from build123d import *
from OCP.BRepFilletAPI import BRepFilletAPI_MakeChamfer

# Parameters (mm, degrees)
SKETCH1_W          = 20.1676
SKETCH1_H          = 40.2082
EXTRUDE1_DEPTH     = 26.4668
SKETCH2_W          = 20.1676
SKETCH2_H          = 40.2082
EXTRUDE2_DEPTH     = 2.4892
SKETCH3_W          = 20.1676
SKETCH3_H          = 40.2082
EXTRUDE3_DEPTH     = 4.445
SKETCH11_W         = 20.1676
SKETCH11_H         = 0.2667
CUT_EXTRUDE2_DEPTH = 4.445
EXTRUDE4_DEPTH     = 2.38125
SKETCH5_R          = 7.62
EXTRUDE5_DEPTH     = 2.57175
CHAMFER1_SIZE      = 2.54
CHAMFER1_SIZE2     = 1.466469684
EXTRUDE6_DEPTH     = 0.635
SKETCH8_R          = 2.778125
EXTRUDE7_DEPTH     = 3.4544
CHAMFER2_SIZE      = 2.54
CHAMFER2_SIZE2     = 1.466469684
FILLET1_R          = 1.016
FILLET2_R          = 1.524
SKETCH9_W          = 6.35
SKETCH9_H          = 2.54
EXTRUDE8_DEPTH     = 2.38125
SKETCH10_W         = 5.08
SKETCH10_H         = 1.27
CUT_EXTRUDE1_DEPTH = 2.38125


with BuildPart() as part:
    # Sketch1 → Extrude1 (new body)
    with BuildSketch(Plane(origin=(0, 0, 0), x_dir=(1, 0, 0), z_dir=(0, 1, 0))):
        with Locations((0, -9.9187)):
            Rectangle(SKETCH1_W, SKETCH1_H)
    extrude(amount=EXTRUDE1_DEPTH)

    # Sketch2 → Extrude2 (add)
    with BuildSketch(Plane(origin=(0, 26.4668, 0), x_dir=(-1, 0, 0), z_dir=(0, 1, 0))):
        with Locations((0, 9.9187)):
            Rectangle(SKETCH2_W, SKETCH2_H)
        with BuildLine():
            ThreePointArc((6.7183, -15.285015296), (5.0673, -11.7348), (3.4163, -15.285015296))
            Line((3.4163, -15.285015296), (3.4163, -16.51))
            Line((3.4163, -16.51), (-3.4163, -16.51))
            Line((-3.4163, -16.51), (-3.4163, -15.285015296))
            ThreePointArc((-3.4163, -15.285015296), (-5.0673, -11.7348), (-6.7183, -15.285015296))
            Line((-6.7183, -15.285015296), (-6.7183, -16.51))
            Line((-6.7183, -16.51), (-10.0838, -16.51))
            Line((-10.0838, -16.51), (-10.0838, -10.1854))
            Line((-10.0838, -10.1854), (10.0838, -10.1854))
            Line((10.0838, -10.1854), (10.0838, -16.51))
            Line((10.0838, -16.51), (6.7183, -16.51))
            Line((6.7183, -16.51), (6.7183, -15.285015296))
        make_face()
        with BuildLine():
            ThreePointArc((-6.7183, 35.122415296), (-5.0673, 31.5722), (-3.4163, 35.122415296))
            Line((-3.4163, 35.122415296), (-3.4163, 36.3474))
            Line((-3.4163, 36.3474), (3.4163, 36.3474))
            Line((3.4163, 36.3474), (3.4163, 35.122415296))
            ThreePointArc((3.4163, 35.122415296), (5.0673, 31.5722), (6.7183, 35.122415296))
            Line((6.7183, 35.122415296), (6.7183, 36.3474))
            Line((6.7183, 36.3474), (10.0838, 36.3474))
            Line((10.0838, 36.3474), (10.0838, 30.0228))
            Line((10.0838, 30.0228), (-10.0838, 30.0228))
            Line((-10.0838, 30.0228), (-10.0838, 36.3474))
            Line((-10.0838, 36.3474), (-6.7183, 36.3474))
            Line((-6.7183, 36.3474), (-6.7183, 35.122415296))
        make_face()
    extrude(amount=EXTRUDE2_DEPTH)

    # Sketch3 → Extrude3 (add)
    with BuildSketch(Plane(origin=(0, 28.956, 0), x_dir=(-1, 0, 0), z_dir=(0, 1, 0))):
        with Locations((0, 9.9187)):
            Rectangle(SKETCH3_W, SKETCH3_H)
    extrude(amount=EXTRUDE3_DEPTH)

    # Sketch11 → Cut-Extrude2 (cut)
    with BuildSketch(Plane(origin=(0, 33.401, 0), x_dir=(1, 0, 0), z_dir=(0, 1, 0))):
        with Locations((0, 10.05205)):
            Rectangle(SKETCH11_W, SKETCH11_H)
        with Locations((0, -29.88945)):
            Rectangle(SKETCH11_W, SKETCH11_H)
    extrude(amount=-CUT_EXTRUDE2_DEPTH, mode=Mode.SUBTRACT)

    # Sketch4 → Extrude4 (add)
    with BuildSketch(Plane(origin=(0, 33.401, 0), x_dir=(-1, 0, 0), z_dir=(0, 1, 0))):
        with BuildLine():
            Line((9.652, 2.228840954), (9.652, 23.6728))
            Line((9.652, 23.6728), (4.655896906, 23.6728))
            ThreePointArc((4.655896906, 23.6728), (0, 26.7208), (-4.655896906, 23.6728))
            Line((-4.655896906, 23.6728), (-9.652, 23.6728))
            Line((-9.652, 23.6728), (-9.652, 2.228840954))
            ThreePointArc((-9.652, 2.228840954), (0, -9.906), (9.652, 2.228840954))
        make_face()
    extrude(amount=EXTRUDE4_DEPTH)

    # Sketch5 → Extrude5 (add)
    with BuildSketch(Plane(origin=(0, 35.78225, 0), x_dir=(-1, 0, 0), z_dir=(0, 1, 0))):
        with Locations(Location((0, 0, 0), (0, 0, 270))):
            Circle(SKETCH5_R)
    extrude(amount=EXTRUDE5_DEPTH)

    # Chamfer1
    chamfer1_edges = [part.edges().sort_by_distance(p)[0] for p in [
        (0, 38.354, 7.62),
    ]]
    chamfer1_side = [part.faces().sort_by_distance(p)[0] for p in [
        (0, 38.354, 0),
    ]]
    chamfer(chamfer1_edges, length=CHAMFER1_SIZE, length2=CHAMFER1_SIZE2, reference=chamfer1_side[0])

    # Sketch7 → Extrude6 (add, symmetric)
    with BuildSketch(Plane(origin=(0, 0, 0), x_dir=(0, 0, -1), z_dir=(1, 0, 0))):
        Polygon((15.2527, 28.956), (12.7127, 30.734), (9.9187, 30.734), (9.9187, 28.956), align=None)
    extrude6 = extrude(amount=EXTRUDE6_DEPTH, both=True)

    # Mirror1: Extrude6 across plane
    add(extrude6.mirror(Plane(origin=(0, 0, 9.9187), x_dir=(1, 0, 0), z_dir=(0, 0, -1))))

    # Sketch8 → Extrude7 (add)
    with BuildSketch(Plane(origin=(0, 38.354, 0), x_dir=(-1, 0, 0), z_dir=(0, 1, 0))):
        with Locations(Location((0, 0, 0), (0, 0, 270))):
            Circle(SKETCH8_R)
    extrude(amount=EXTRUDE7_DEPTH)

    # Chamfer2: one chamfer whose edges measure the first distance from different faces: ONE call of the kernel's chamfer builder (chamfer() names one face for all edges)
    chamfer2_edges_1 = [part.edges().sort_by_distance(p)[0] for p in [
        (0, 0, -10.1854),
    ]]
    chamfer2_side_1 = [part.faces().sort_by_distance(p)[0] for p in [
        (0, 13.2334, -10.1854),
    ]]
    chamfer2_edges_2 = [part.edges().sort_by_distance(p)[0] for p in [
        (0, 0, 30.0228),
    ]]
    chamfer2_side_2 = [part.faces().sort_by_distance(p)[0] for p in [
        (0, 13.2334, 30.0228),
    ]]
    chamfer2 = BRepFilletAPI_MakeChamfer(part.part.solid().wrapped)
    for e in chamfer2_edges_1:
        chamfer2.Add(CHAMFER2_SIZE, CHAMFER2_SIZE2, e.wrapped, chamfer2_side_1[0].wrapped)  # the first distance lies on this face
    for e in chamfer2_edges_2:
        chamfer2.Add(CHAMFER2_SIZE, CHAMFER2_SIZE2, e.wrapped, chamfer2_side_2[0].wrapped)  # the first distance lies on this face
    add(Compound.cast(chamfer2.Shape()), mode=Mode.REPLACE)

    # Fillet1
    fillet1_edges = [part.edges().sort_by_distance(p)[0] for p in [
        (10.0838, 0, 9.9187),
        (10.0838, 1.27, -9.452165158),
        (10.0838, 14.5034, -10.1854),
        (0, 0, -8.718930316),
        (0, 2.54, -10.1854),
        (-10.0838, 14.5034, -10.1854),
        (-10.0838, 1.27, -9.452165158),
        (10.0838, 14.5034, 30.0228),
        (10.0838, 1.27, 29.289565158),
        (0, 2.54, 30.0228),
        (-10.0838, 0, 9.9187),
        (0, 0, 28.556330316),
        (-10.0838, 1.27, 29.289565158),
        (-10.0838, 14.5034, 30.0228),
        (10.0838, 31.1785, 29.7561),
        (-10.0838, 31.1785, 29.7561),
        (10.0838, 31.1785, -9.9187),
        (-10.0838, 31.1785, -9.9187),
    ]]
    fillet(fillet1_edges, radius=FILLET1_R)

    # Fillet2
    fillet2_edges = [part.edges().sort_by_distance(p)[0] for p in [
        (-10.0838, 27.7114, 36.3474),
        (10.0838, 27.7114, 36.3474),
        (-10.0838, 27.7114, -16.51),
        (10.0838, 27.7114, -16.51),
    ]]
    fillet(fillet2_edges, radius=FILLET2_R)

    # Sketch9 → Extrude8 (add)
    with BuildSketch(Plane(origin=(0, 0, -10.1854), x_dir=(-1, 0, 0), z_dir=(0, 0, -1))):
        with Locations((0, 4.318)):
            Rectangle(SKETCH9_W, SKETCH9_H)
    extrude(amount=EXTRUDE8_DEPTH)

    # Sketch10 → Cut-Extrude1 (cut)
    with BuildSketch(Plane(origin=(0, 0, -12.56665), x_dir=(-1, 0, 0), z_dir=(0, 0, -1))):
        with Locations((0, 4.318)):
            Rectangle(SKETCH10_W, SKETCH10_H)
    extrude(amount=-CUT_EXTRUDE1_DEPTH, mode=Mode.SUBTRACT)


solid = part.part
Can you work these out from the model? Positions are in its coordinate system, mm. A direction names the side the tool comes from. Coordinates: 2 decimals unless noted, no trailing zeros. Loops run counter-clockwise (first coordinate to the right, second up) from the corner with the lowest first, then second, coordinate; pieces in that order, holes last. Notation, with made-up numbers: M -26.75,88 L 6.25,88 A34 cw 6.25,125 Z; hole C 70.5,7.25 d4. An arc over 180 degrees is marked long. Return JSON: item names as keys, results as strings. Group by question number.
Item 1: Imagine slicing it at A-A (z = 0). Please give me the cut outline in (x, y), and give its area (3 significant figures).
Item 2: Thinking about a two-plate mould opening in Y: for faces 5 (the flat face through (0, 4, -10.185)), 6 (the flat face through (0, 0, 10)), 7 (the flat face through (0, 28, -16.51)), which applies, released by +Y, released by -Y, zero draft, split by the parting line, or undercut?
Item 3: If I drill on L1, parallel to X at y = 27, z = 32.5; L2, parallel to X at y = 28, z = 32; L3, parallel to Y at x = 4.75, z = 27.5, over which ranges is the centre line in solid material (lowest first)? Write a range as from..to.
Item 4: I'm going to push flat-ended pins straight in: pin 1 Ø7 at (x, z) = (5.07, 33.73) entering from -Y; pin 2 Ø8.5 at (x, z) = (4.5, -14) entering from +Y; pin 3 Ø1.9 at (x, z) = (-1, -11.5) entering from -Y; pin 4 Ø2.5 at (x, z) = (-5.07, -13.89) entering from -Y. Where does each tip first touch, or does it pass through?
Item 5: Imagine slicing it at B-B (y = 24). Please give me the cut outline in (x, z).
Item 6: On a 3-axis mill with a long thin cutter (end or side, diameter ignored), from which of +Z, -Z, +X, -X, +Y, -Y can I reach the whole of each face in a straight line? I mean faces 1 (the flat face through (0, 3.683, -11)), 2 (the cylindrical face through (-2.343, 40.057, -1.494)), 3 (the flat face through (7, 35, 23.673)), 4 (the flat face through (-0.635, 30, 32)). Say none if no direction works.
Item 7: Imagine slicing it at C-C (z = 12.5). Please give me the cut outline in (x, y).
Verdict:
{
 "1": {"outline": "M -10.08,1.02 A1.02 ccw -9.07,0 L 9.07,0 A1.02 ccw 10.08,1.02 L 10.08,33.4 L 9.91,33.4 L 9.91,35.78 L 7.62,35.78 L 7.62,36.89 L 5.08,38.35 L 2.78,38.35 L 2.78,41.81 L -2.78,41.81 L -2.78,38.35 L -5.08,38.35 L -7.62,36.89 L -7.62,35.78 L -9.91,35.78 L -9.91,33.4 L -10.08,33.4 Z", "area": "775 mm^2"},
 "2": {"face 5": "undercut", "face 6": "released by -Y", "face 7": "zero draft"},
 "3": {"L1": "x = -10.08..-6.84, -3.29..3.29, 6.84..10.08", "L2": "x = -10.08..-6.36, -3.78..3.78, 6.36..10.08", "L3": "y = 0..33.4"},
 "4": {"pin 1": "stops at y = 26.47", "pin 2": "stops at y = 33.4", "pin 3": "stops at y = 3.05", "pin 4": "passes through"},
 "5": {"outline": "M -10.08,-9.17 A1.02 ccw -9.07,-10.19 L 9.07,-10.19 A1.02 ccw 10.08,-9.17 L 10.08,29.01 A1.02 ccw 9.07,30.02 L -9.07,30.02 A1.02 ccw -10.08,29.01 Z"},
 "6": {"face 1": "-Z", "face 2": "+Y", "face 3": "+Z, +X, +Y", "face 4": "+Z, -X, +Y"},
 "7": {"outline": "M -10.08,1.02 A1.02 ccw -9.07,0 L 9.07,0 A1.02 ccw 10.08,1.02 L 10.08,33.4 L 9.65,33.4 L 9.65,35.78 L -9.65,35.78 L -9.65,33.4 L -10.08,33.4 Z"}
}
